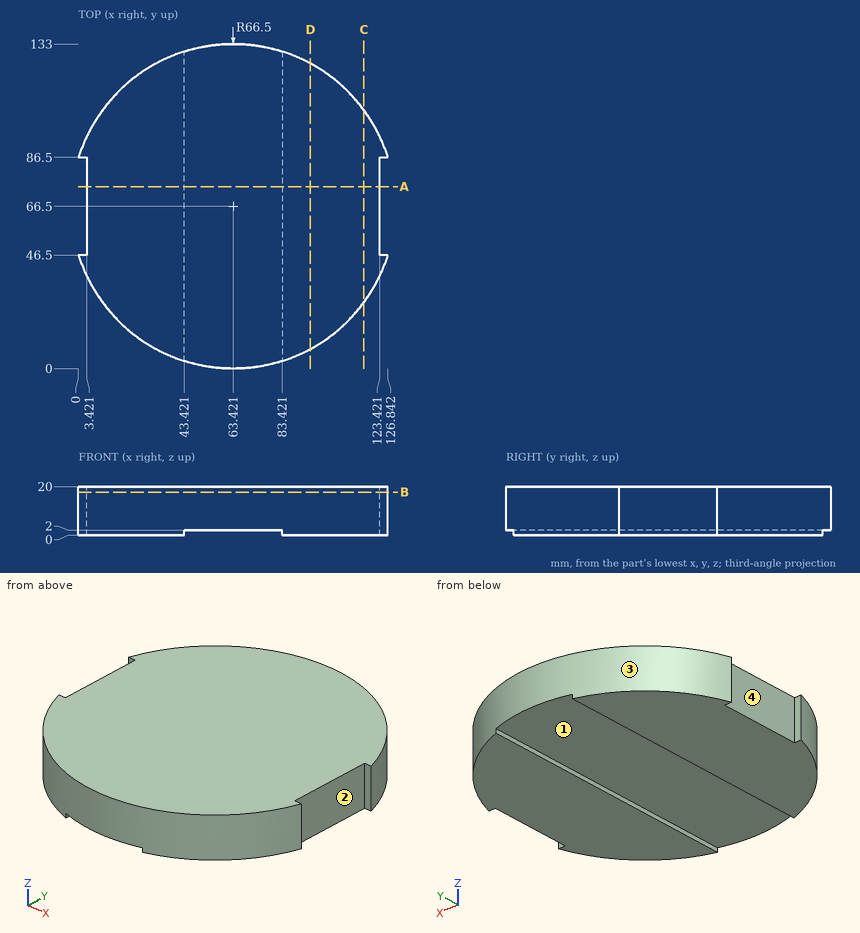
The drawing under review shows one solid part. Ordinate dimensions are in mm from its lowest x, y, z. Give positions to 0.01 mm unless a question says otherwise; leave off trailing zeros. Write each loop counter-clockwise with the first axis right and the second up, starting at its lowest first coordinate (ties: lowest second). Pieces come first, ordered by that corner, then holes. Notation, with made-up numbers: (84, 42) -> (99, 42) arc R4 cw to (99, 46) -> close; hole circle Ø2 at (-36, 24). An arc over 180 degrees is marked (long way). Use CSV: the item, a comma, the result in double quotes.
Q1. To check wall thickness, follow probe 1 along X at (y, z) = (78, 3.75); probe 2 along Z at (x, y) = (51, 60.5); probe 3 along Y at (x, z) = (49, 7). State the ranges of each line that lie inside material, in increasing order. Write a range as [from, to].
Conclusion:
probe 1,"[3.42, 123.42]"
probe 2,"[2, 20]"
probe 3,"[1.58, 131.42]"
Q2. Take a section at A-A, the plane y = 74.5. Write out the cut boundary in (x, z).
Conclusion:
outline,"(3.42, 0) -> (43.42, 0) -> (43.42, 2) -> (83.42, 2) -> (83.42, 0) -> (123.42, 0) -> (123.42, 20) -> (3.42, 20) -> close"
Q3. Take a section at D-D, the plane x = 95. Write out the cut boundary in (y, z), then the cut area to 3 significant figures.
Conclusion:
outline,"(7.98, 0) -> (125.02, 0) -> (125.02, 20) -> (7.98, 20) -> close"
area,"2,340 mm2"
Q4. For P1, Ø4, axis at x = 80, z = 9.5, coming from the +Y side; P2, Ø1.6, axis at y = 66.5, z = 1.5, coming from the +X side; P3, Ø12, axis at x = 65.5, y = 93, coming from the -Z side, all flat-tipped, find the tip position at first contact; note any pin that passes through.
Conclusion:
P1,"y = 131.38"
P2,"x = 123.42"
P3,"z = 2"
Q5. Mouldability with a two-part tool opening along Y and no side actions: class the marked faces 1, 2, 3 and 4 as pulls with the +Y half, pulls with the -Y half, needs draft (parallel to the pull), parting line crosses it, or undercut.
Conclusion:
face 1,"needs draft"
face 2,"undercut"
face 3,"pulls with the +Y half"
face 4,"undercut"
Q6. Take a section at C-C, the plane x = 117. Write out the cut boundary in (y, z), then the cut area to 3 significant figures.
Conclusion:
outline,"(27.11, 0) -> (105.89, 0) -> (105.89, 20) -> (27.11, 20) -> close"
area,"1,580 mm2"
Q7. Take a section at B-B, the plane z = 17.75. Write out the cut boundary in (x, y), then the cut area to 3 significant figures.
Conclusion:
outline,"(0, 46.5) arc R66.5 ccw to (126.84, 46.5) -> (123.42, 46.5) -> (123.42, 86.5) -> (126.84, 86.5) arc R66.5 ccw to (0, 86.5) -> (3.42, 86.5) -> (3.42, 46.5) -> close"
area,"13,500 mm2"
